For this review, use the dimensioned drawing (mm, ordinates from the lowest corner) and the shaded views. Give positions to 0.01 mm unless a question says otherwise; leave off trailing zeros. Order: outer loops, then holes, each group sorted by start corner. A loop starts at its lowest first (then second) coordinate and runs counter-clockwise, first axis right, second up.
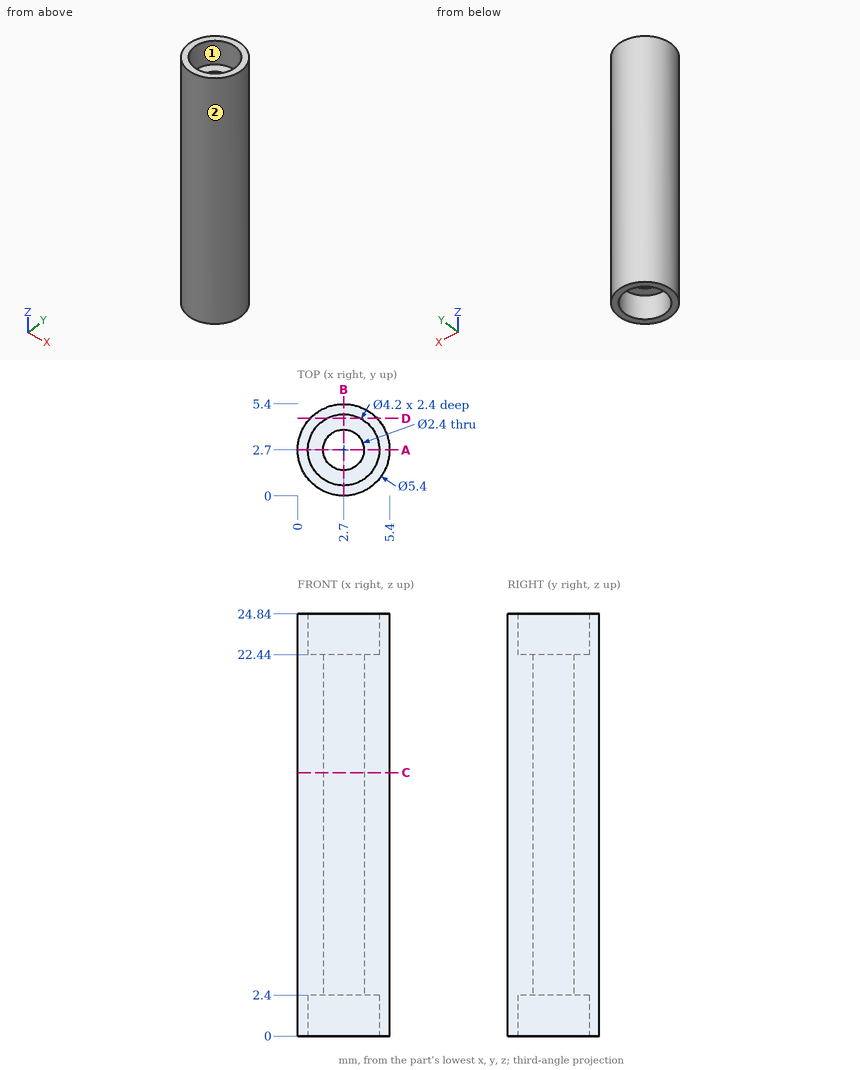
1. For pin 1 (2.5 mm diameter, centred on x = 2.7, y = 2.7, fed in from +Z); pin 2 (2 mm diameter, centred on x = 1, z = 6, fed in from -Y), all flat-tipped, find the tip position at first contact; note any pin that passes through.
Recorded:
pin 1: stops at z = 22.44
pin 2: stops at y = 0.09
2. Take a section at C-C (z = 15.5). State the section outline as (x, y) points.
Recorded:
outline: circle Ø5.4 at (2.7, 2.7); hole circle Ø2.4 at (2.7, 2.7)
3. Take a section at A-A (y = 2.7). State the section outline as (x, z) points, then the cut area to 3 significant figures.
Recorded:
outline: (0, 0) - (0.6, 0) - (0.6, 2.4) - (1.5, 2.4) - (1.5, 22.44) - (0.6, 22.44) - (0.6, 24.84) - (0, 24.84) - close; (3.9, 2.4) - (4.8, 2.4) - (4.8, 0) - (5.4, 0) - (5.4, 24.84) - (4.8, 24.84) - (4.8, 22.44) - (3.9, 22.44) - close
area: 65.9 mm2
4. For line 1 along X through (y, z) = (2.7, 0.85); line 2 along Z through (x, y) = (3, 1); line 3 along X through (y, z) = (3.2, 14.75), list the stretches that pass through material, from the lowest coordinate up.
Recorded:
line 1: x = 0 to 0.6, 4.8 to 5.4
line 2: z = 2.4 to 22.44
line 3: x = 0.05 to 1.61, 3.79 to 5.35
5. Draft analysis for pull direction X (two halves, no side actions). For the marked faces 1 and 2, state which applies: pulls with the +X half, pulls with the -X half, needs draft (parallel to the pull), parting line crosses it, or undercut.
Recorded:
face 1: undercut
face 2: parting line crosses it
6. Take a section at D-D (y = 4.55). State the section outline as (x, z) points.
Recorded:
outline: (0.73, 0) - (1.71, 0) - (1.71, 2.4) - (3.69, 2.4) - (3.69, 0) - (4.67, 0) - (4.67, 24.84) - (3.69, 24.84) - (3.69, 22.44) - (1.71, 22.44) - (1.71, 24.84) - (0.73, 24.84) - close
